```python
from build123d import *

# Parameters (mm, degrees)
F0_R     = 12
F0_R_2   = 1.75
F0_R_3   = 4
F1_DEPTH = 8
F0_R_4   = 6.75
F2_DEPTH = 2
F3_R     = 8
F4_R     = 1.5
F5_DEPTH = 10


with BuildPart() as f1:
    # F0 (on Top) → F1 (new body)
    with BuildSketch(Plane.XY):
        Polygon((30.25, 0), (20.75, 0), (20.75, -7.8), (0, -7.8), (-4, -7.8), (-4, -53), (0, -53), (51, -53), (51, -7.8), (30.25, -7.8), align=None)
        with Locations((11, -37.5)):
            Circle(F0_R, mode=Mode.SUBTRACT)
        with Locations((33, -46.5)):
            Circle(F0_R_2, mode=Mode.SUBTRACT)
        with Locations((33, -37.5)):
            Circle(F0_R_3, mode=Mode.SUBTRACT)
        with Locations((33, -28.5)):
            Circle(F0_R_2, mode=Mode.SUBTRACT)
    extrude(amount=F1_DEPTH)

    # F0 (on Top) → F2 (join)
    with BuildSketch(Plane.XY):
        with Locations((11, -37.5)):
            Circle(F0_R)
        with Locations((11, -37.5)):
            Circle(F0_R_4, mode=Mode.SUBTRACT)
    extrude(amount=F2_DEPTH)

    # F3
    f3_edges = [f1.edges().sort_by_distance(p)[0] for p in [
        (-4, -53, 4),
        (51, -53, 4),
    ]]
    fillet(f3_edges, radius=F3_R)

    # F4 (on face) → F5 (cut)
    with BuildSketch(Plane(origin=(0, -7.8, 0), x_dir=(-1, 0, 0), z_dir=(0, 1, 0))):
        with Locations((-41.25, 4)):
            Circle(F4_R)
        with Locations((-9.75, 4)):
            Circle(F4_R)
    extrude(amount=-F5_DEPTH, mode=Mode.SUBTRACT)


solid = f1.part
```
Verification items for the finished model (mm, model axes). A direction names the side the tool comes from. Coordinates: 2 decimals unless noted, no trailing zeros. Write each loop counter-clockwise with the first axis right and the second up, starting at its lowest first coordinate (ties: lowest second). Pieces come first, ordered by that corner, then holes. Notation, with made-up numbers: (23.5, 35.5) - (41.5, 35.5) arc R15 cw to (41.5, 61.5) - close; hole circle Ø5 at (-29.75, -13.75). An arc over 180 degrees is marked (long way). One line per question, with ' | ' between items. Start each with the question number.
1. Section check A-A (y = -37.5). Enter the section's corners in (x, z), plus the area to 3 significant figures.
2. Gauge pin test, flat ends, axial feed: P1, Ø3, axis at x = 33, y = -46.5, coming from the +Z side; P2, Ø2.5, axis at x = 41, z = 4.5, coming from the +Y side; P3, Ø12, axis at x = 8, y = -38, coming from the +Z side. Record the tip position at first contact, or that the pin passes through.
3. Access from +Z, -Z, +X, -X, +Y, -Y to the whole of each face (thin tool, end or side, straight path). Record for faces 1 (the cylindrical face through (42.75, -12.73, 4.07)), 2 (the flat face through (9, -7.8, 2)), 3 (the cylindrical face through (9.44, -25.6, 4.96)), 4 (the flat face through (30.25, -4, 4)).
4. Material ranges on line 1 along Y through (x, z) = (11.5, 2.75); line 2 along X through (y, z) = (-45, 5.5); line 3 along Y through (x, z) = (33, 2), recorded low to high.
5. Section check B-B (z = 6.5). Enter the section's corners in (x, y), plus the area to 3 significant figures.
6. Section check C-C (x = 33). Enter the section's corners in (y, z).
7. Draft check along Z on faces 5 (the flat face through (23, -26, 8)), 6 (the cylindrical face through (32.479, -33.534, 3.944)), 7 (the flat face through (41, -17.8, 4)). Enter one of: released by +Z, released by -Z, zero draft, split by the parting line, or undercut.
8. Section check D-D (x = 41.25). Enter the section's corners in (y, z), plus the area to 3 significant figures.
Computed values:
1) outline: (-4, 0) - (4.25, 0) - (4.25, 2) - (-1, 2) - (-1, 8) - (-4, 8) - close; (17.75, 0) - (29, 0) - (29, 8) - (23, 8) - (23, 2) - (17.75, 2) - close; (37, 0) - (51, 0) - (51, 8) - (37, 8) - close | area: 205 mm²
2) P1: through | P2: y = -7.8 | P3: z = 2
3) face 1: +Y | face 2: +Z, -Z, -X, +Y | face 3: +Z | face 4: +Z, -Z, +X, +Y
4) line 1: -53 to -49.49, -25.51 to -7.8 | line 2: -4 to 1.63, 20.37 to 32.1, 33.9 to 51 | line 3: -53 to -48.25, -44.75 to -41.5, -33.5 to -30.25, -26.75 to -7.8
5) outline: (-4, -45) arc R8 ccw to (4, -53) - (43, -53) arc R8 ccw to (51, -45) - (51, -7.8) - (30.25, -7.8) - (30.25, 0) - (20.75, 0) - (20.75, -7.8) - (-4, -7.8) - close; hole circle Ø24 at (11, -37.5); hole circle Ø8 at (33, -37.5); hole circle Ø3.5 at (33, -46.5); hole circle Ø3.5 at (33, -28.5) | area: 2,010 mm²
6) outline: (-53, 0) - (-48.25, 0) - (-48.25, 8) - (-53, 8) - close; (-44.75, 0) - (-41.5, 0) - (-41.5, 8) - (-44.75, 8) - close; (-33.5, 0) - (-30.25, 0) - (-30.25, 8) - (-33.5, 8) - close; (-26.75, 0) - (-7.8, 0) - (-7.8, 8) - (-26.75, 8) - close
7) face 5: released by +Z | face 6: zero draft | face 7: undercut
8) outline: (-53, 0) - (-7.8, 0) - (-7.8, 2.5) - (-17.8, 2.5) - (-17.8, 5.5) - (-7.8, 5.5) - (-7.8, 8) - (-53, 8) - close | area: 332 mm²
